Input: dimensioned drawing with shaded views. Units: mm. Origin: part minimum x, y, z. Coordinates: 2 decimals unless noted, no trailing zeros. Order: outer loops, then holes, each group sorted by start corner. A loop starts at its lowest first (then second) coordinate and runs counter-clockwise, first axis right, second up. Notation, with made-up numbers: (63, 80) -> (96, 80) arc R12 cw to (96, 92) -> close; hole circle Ø11 at (21, -5.5). An arc over 180 degrees is marked (long way). Answer as CSV lines item,"result".
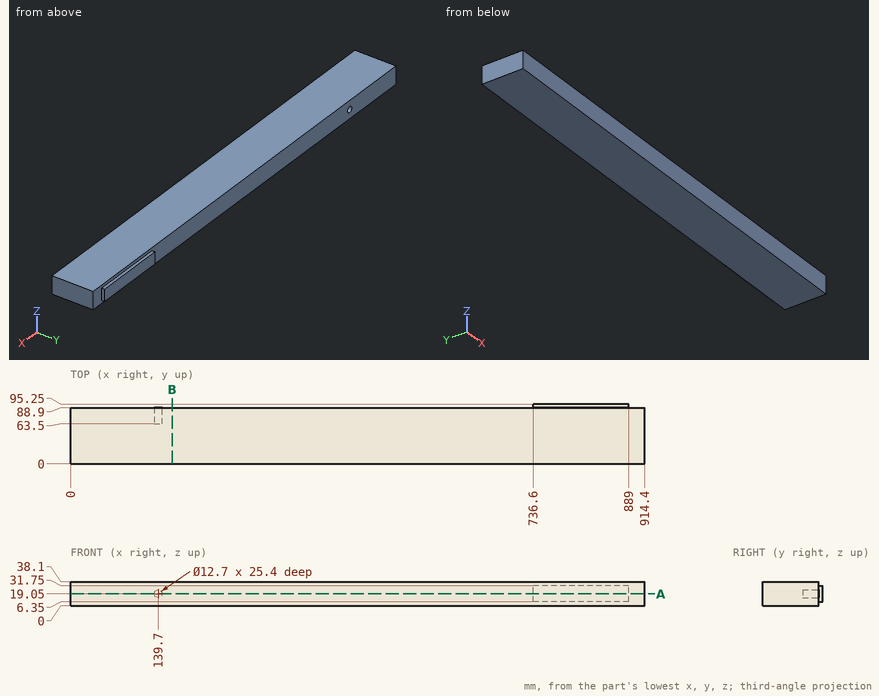
1. Contact query for flat-ended pins moving along their axis: pin 1 (7 mm diameter, centred on y = 93, z = 15, fed in from +X); pin 2 (6.5 mm diameter, centred on x = 140.5, z = 16, fed in from +Y); pin 3 (1.9 mm diameter, centred on x = 845.5, y = 92.5, fed in from -Z). Output: stop coordinate, or through.
Findings:
pin 1,"stops at x = 889"
pin 2,"stops at y = 88.9"
pin 3,"stops at z = 6.35"
2. Cut plane A-A (z = 19.05). Return the cut outline in (x, y), plus the area to 3 significant figures.
Findings:
outline,"(0, 0) -> (914.4, 0) -> (914.4, 88.9) -> (889, 88.9) -> (889, 95.25) -> (736.6, 95.25) -> (736.6, 88.9) -> (146.05, 88.9) -> (146.05, 63.5) -> (133.35, 63.5) -> (133.35, 88.9) -> (0, 88.9) -> close"
area,"81,900 mm2"
3. Ray query, line 1 along Z through (x, y) = (139.7, 71); line 2 along Y through (x, z) = (318, 25). Return the intervals inside material, ascending.
Findings:
line 1,"z = 0 to 12.7, 25.4 to 38.1"
line 2,"y = 0 to 88.9"
4. Cut plane B-B (x = 162). Return the cut outline in (y, z).
Findings:
outline,"(0, 0) -> (88.9, 0) -> (88.9, 38.1) -> (0, 38.1) -> close"
